CAD build for the part. Positions are in the model's coordinates, mm. A direction names the side the tool comes from. Round coordinates to 2 decimals unless told otherwise and drop trailing zeros. Loops run counter-clockwise (first coordinate to the right, second up) from the corner with the lowest first, then second, coordinate; pieces in that order, holes last. Notation, with made-up numbers: M 89.25,38.25 L 94.25,38.25 A29 cw 94.25,73.25 Z; hole C 83.5,12 d8. An arc over 180 degrees is marked long. Use a Markdown table: item, result. Add a question column.
(1) Band-saw the part on C-C, the plane x = -12. Write the cut outline in (y, z) (3 decimals).
(2) Flat gauge pins, fed straight in: P1, Ø12, axis at x = -22, y = 17, coming from the +Z side; P2, Ø4, axis at x = -14.5, z = -1.5, coming from the -Y side (3 decimals); P3, Ø0.8, axis at y = -52.5, z = -1.5, coming from the -X side; P4, Ø2, axis at y = -51.5, z = -2, coming from the +X side. Where does each tip first touch, or does it go through?
(3) Two-plate mould, pull along Y, no slides. Class faces 4 (the face through (-39.37, -1, 3)), 5 (the face through (-37.105, -49.261, 2.504)): released by +Y, released by -Y, zero draft, split by the parting line, or undercut.
(4) Which spindle directions (+Z, -Z, +X, -X, +Y, -Y) get a long thin tool onto all of the face, cutting with end or side? Do faces 1 (the face through (14.336, 37.922, 4.83)), 2 (the face through (-1, 1, 5.08)), 3 (the face through (-1, 1, 4.572)). Say none if no direction does.
(5) Band-saw the part on B-B, the plane y = 10. Write the cut outline in (x, z), and give its area (3 significant figures).
(6) Band-saw the part on A-A, the plane x = 12. Write the cut outline in (y, z) (3 decimals), and give its area (3 significant figures).
(7) Wall check: L1, parallel to Y at x = -17, z = 4.75 (3 decimals); L2, parallel to X at y = -15.5, z = 5; L3, parallel to X at y = 38.5, z = 2.75. Give the ranges that are in metal, low to high.
from build123d import *

# Parameters (mm, degrees)
BOSS_EXTRUDE1_DEPTH = 5.588
CUT_EXTRUDE1_DEPTH  = 0.508
SHELL2_T            = -0.508
SKETCH3_R           = 5.969
CUT_EXTRUDE2_DEPTH  = 0.508
SKETCH5_W           = 2.54
SKETCH5_H           = 0.508
BOSS_EXTRUDE2_DEPTH = 76.708
SKETCH7_R           = 1.27
BOSS_EXTRUDE3_DEPTH = 76.708
CUT_EXTRUDE3_DEPTH  = 79.74
SKETCH9_R           = 1.016
CUT_EXTRUDE4_DEPTH  = 79.74
SKETCH10_W          = 7.112
SKETCH10_H          = 2.032
SKETCH10_W_2        = 12.7
CUT_EXTRUDE5_DEPTH  = 9.382
SKETCH11_W          = 10.616681579
SKETCH11_H          = 2.54
SKETCH11_W_2        = 10.870681579
CUT_EXTRUDE6_DEPTH  = 3.5400001
SKETCH12_W          = 7.112
SKETCH12_H          = 2.54
CUT_EXTRUDE7_DEPTH  = 3.54


with BuildPart() as part:
    # Sketch1 → Boss-Extrude1 (new body)
    with BuildSketch(Plane.XY):
        with BuildLine():
            Line((-33.02, 51.435), (33.02, 51.435))
            ThreePointArc((33.02, 51.435), (37.510128061, 49.575128061), (39.37, 45.085))
            Line((39.37, 45.085), (39.37, -45.085))
            ThreePointArc((39.37, -45.085), (37.510128061, -49.575128061), (33.02, -51.435))
            Line((33.02, -51.435), (-33.02, -51.435))
            ThreePointArc((-33.02, -51.435), (-37.510128061, -49.575128061), (-39.37, -45.085))
            Line((-39.37, -45.085), (-39.37, 45.085))
            ThreePointArc((-39.37, 45.085), (-37.510128061, 49.575128061), (-33.02, 51.435))
        make_face()
    extrude(amount=BOSS_EXTRUDE1_DEPTH)

    # Sketch2 → Cut-Extrude1 (cut)
    with BuildSketch(Plane.XY.offset(5.588)):
        with BuildLine():
            Line((-29.972, -48.387), (29.972, -48.387))
            ThreePointArc((29.972, -48.387), (34.462128061, -46.527128061), (36.322, -42.037))
            Line((36.322, -42.037), (36.322, 42.037))
            ThreePointArc((36.322, 42.037), (34.462128061, 46.527128061), (29.972, 48.387))
            Line((29.972, 48.387), (-29.972, 48.387))
            ThreePointArc((-29.972, 48.387), (-34.462128061, 46.527128061), (-36.322, 42.037))
            Line((-36.322, 42.037), (-36.322, -42.037))
            ThreePointArc((-36.322, -42.037), (-34.462128061, -46.527128061), (-29.972, -48.387))
        make_face()
    extrude(amount=-CUT_EXTRUDE1_DEPTH, mode=Mode.SUBTRACT)

    # Shell2
    shell2_openings = [part.faces().sort_by_distance(p)[0] for p in [
        (0, 0, 0),
    ]]
    offset(amount=SHELL2_T, openings=shell2_openings, kind=Kind.INTERSECTION)

    # Sketch3 → Cut-Extrude2 (cut)
    with BuildSketch(Plane.XY.offset(5.08)):
        with Locations((15.113, 32.004)):
            Circle(SKETCH3_R)
    extrude(amount=-CUT_EXTRUDE2_DEPTH, mode=Mode.SUBTRACT)

    # Sketch5 → Boss-Extrude2 (add)
    with BuildSketch(Plane(origin=(39.37, 0, 0), x_dir=(0, 0, -1), z_dir=(1, 0, 0))):
        with Locations((1.27, -51.181)):
            Rectangle(SKETCH5_W, SKETCH5_H)
    extrude(amount=-BOSS_EXTRUDE2_DEPTH)

    # Sketch7 → Boss-Extrude3 (add)
    with BuildSketch(Plane(origin=(39.37, 0, 0), x_dir=(0, 0, -1), z_dir=(1, 0, 0))):
        with Locations((1.524, -52.197)):
            Circle(SKETCH7_R)
    extrude(amount=-BOSS_EXTRUDE3_DEPTH)

    # Sketch8 → Cut-Extrude3 (cut, through all)
    with BuildSketch(Plane(origin=(39.37, 0, 0), x_dir=(0, 0, -1), z_dir=(1, 0, 0))):
        with BuildLine():
            Line((2.54, -50.927), (1.524, -50.927))
            ThreePointArc((1.524, -50.927), (2.091961266, -51.061077467), (2.54, -51.435))
            Line((2.54, -51.435), (2.54, -50.927))
        make_face()
    extrude(amount=-CUT_EXTRUDE3_DEPTH, mode=Mode.SUBTRACT)

    # Sketch9 → Cut-Extrude4 (cut, through all)
    with BuildSketch(Plane(origin=(39.37, 0, 0), x_dir=(0, 0, -1), z_dir=(1, 0, 0))):
        with Locations((1.524, -52.197)):
            Circle(SKETCH9_R)
    extrude(amount=-CUT_EXTRUDE4_DEPTH, mode=Mode.SUBTRACT)

    # Sketch10 → Cut-Extrude5 (cut, through all)
    with BuildSketch(Plane.XY.offset(5.588)):
        with Locations((-13.97, -52.451)):
            Rectangle(SKETCH10_W, SKETCH10_H)
        with Locations((0.254, -52.451)):
            Rectangle(SKETCH10_W, SKETCH10_H)
        with Locations((14.478, -52.451)):
            Rectangle(SKETCH10_W, SKETCH10_H)
        Polygon((39.37, -54.461005148), (39.37, -51.435), (33.02, -51.435), (24.892, -51.435), (24.892, -54.461005148), align=None)
        with Locations((-30.988, -52.451)):
            Rectangle(SKETCH10_W_2, SKETCH10_H)
        with BuildLine():
            Line((-35.508681579, -50.927), (-37.338, -50.927))
            Line((-37.338, -50.927), (-37.338, -51.435))
            Line((-37.338, -51.435), (-33.02, -51.435))
            ThreePointArc((-33.02, -51.435), (-34.29, -51.306703947), (-35.508681579, -50.927))
        make_face()
        with BuildLine():
            Line((39.37, -50.927), (35.508681579, -50.927))
            ThreePointArc((35.508681579, -50.927), (34.29, -51.306703947), (33.02, -51.435))
            Line((33.02, -51.435), (39.37, -51.435))
            Line((39.37, -51.435), (39.37, -50.927))
        make_face()
    extrude(amount=-CUT_EXTRUDE5_DEPTH, mode=Mode.SUBTRACT)

    # Sketch11 → Cut-Extrude6 (cut, through all)
    with BuildSketch(Plane(origin=(0, -50.927, 0), x_dir=(1, 0, 0), z_dir=(0, 1, 0))):
        with Locations((30.20034079, 1.27)):
            Rectangle(SKETCH11_W, SKETCH11_H)
        with Locations((-30.07334079, 1.27)):
            Rectangle(SKETCH11_W_2, SKETCH11_H)
    extrude(amount=-CUT_EXTRUDE6_DEPTH, mode=Mode.SUBTRACT)

    # Sketch12 → Cut-Extrude7 (cut, through all)
    with BuildSketch(Plane(origin=(0, -50.927, 0), x_dir=(1, 0, 0), z_dir=(0, 1, 0))):
        with Locations((14.478, 1.27)):
            Rectangle(SKETCH12_W, SKETCH12_H)
        with Locations((0.254, 1.27)):
            Rectangle(SKETCH12_W, SKETCH12_H)
        with Locations((-13.97, 1.27)):
            Rectangle(SKETCH12_W, SKETCH12_H)
    extrude(amount=-CUT_EXTRUDE7_DEPTH, mode=Mode.SUBTRACT)


solid = part.part
Return value:
| question | item | result |
|---|---|---|
| 1 | outline | M -51.435,0 L -50.927,0 L -50.927,5.08 L -48.895,5.08 L -48.895,4.572 L 48.895,4.572 L 48.895,5.08 L 50.927,5.08 L 50.927,0 L 51.435,0 L 51.435,5.588 L 48.387,5.588 L 48.387,5.08 L -48.387,5.08 L -48.387,5.588 L -51.435,5.588 Z |
| 2 | P1 | z = 5.08 |
| 2 | P2 | y = -51.435 |
| 2 | P3 | through |
| 2 | P4 | x = 24.89 |
| 3 | face 4 | zero draft |
| 3 | face 5 | undercut |
| 4 | face 1 | +Z, -Z |
| 4 | face 2 | +Z |
| 4 | face 3 | -Z |
| 5 | outline | M -39.37,0 L -38.86,0 L -38.86,5.08 L -36.83,5.08 L -36.83,4.57 L 36.83,4.57 L 36.83,5.08 L 38.86,5.08 L 38.86,0 L 39.37,0 L 39.37,5.59 L 36.32,5.59 L 36.32,5.08 L -36.32,5.08 L -36.32,5.59 L -39.37,5.59 Z |
| 5 | area | 45.7 mm^2 |
| 6 | outline | M -51.435,0 L -50.927,0 L -50.927,5.08 L -48.895,5.08 L -48.895,4.572 L 26.911,4.572 L 26.911,5.08 L -48.387,5.08 L -48.387,5.588 L -51.435,5.588 Z; M 37.097,4.572 L 48.895,4.572 L 48.895,5.08 L 50.927,5.08 L 50.927,0 L 51.435,0 L 51.435,5.588 L 48.387,5.588 L 48.387,5.08 L 37.097,5.08 Z |
| 6 | area | 52.8 mm^2 |
| 7 | L1 | -51.435 to -50.927, -48.895 to 48.895, 50.927 to 51.435 |
| 7 | L2 | -39.37 to -38.86, -36.83 to 36.83, 38.86 to 39.37 |
| 7 | L3 | -39.37 to -38.86, 38.86 to 39.37 |
